Geometry: see drawing. Coordinates: mm, zero at the bounding-box minimum. A direction names the side the tool comes from. Round coordinates to 2 decimals unless told otherwise and drop trailing zeros. Write each loop counter-clockwise with the first axis right and the second up, starting at its lowest first coordinate (ties: lowest second). Pieces come first, ordered by that corner, then holes. Notation, with made-up numbers: (1.25, 89.5) -> (27.25, 89.5) arc R28 ccw to (27.25, 112.5) -> close; hole circle Ø1 at (58, 9). An arc over 180 degrees is marked (long way). Write item = value, one per line.
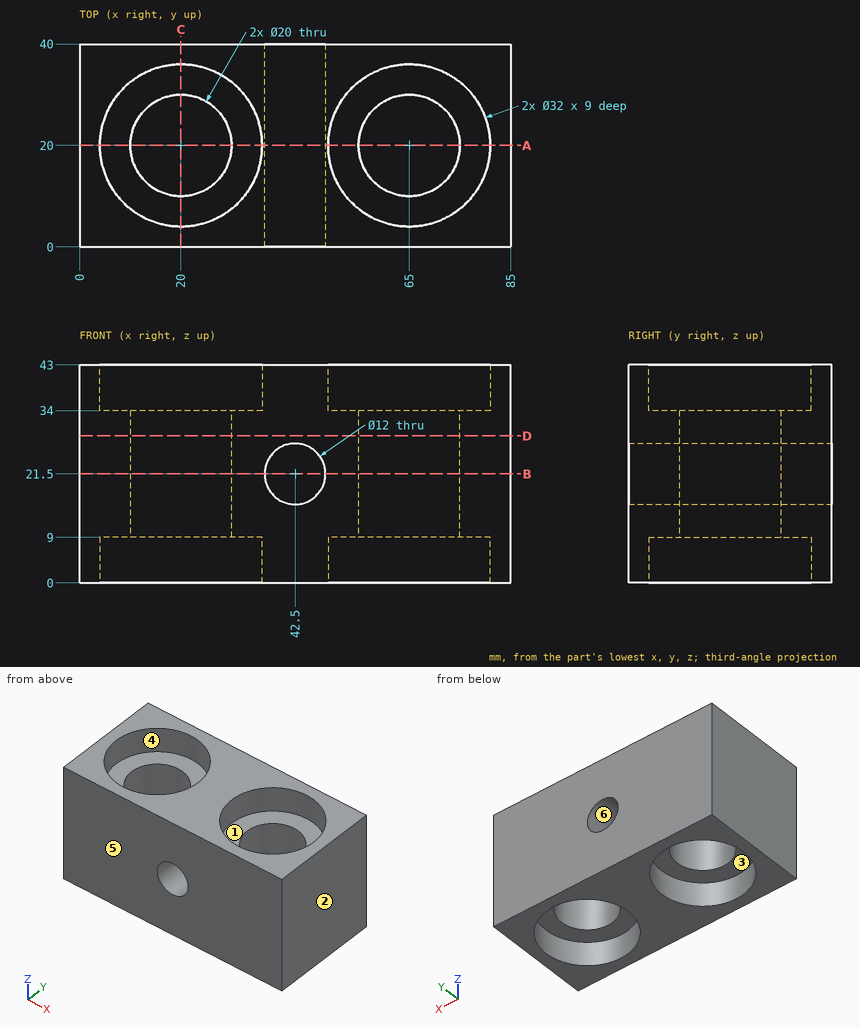
1) Cut plane B-B (z = 21.5). Return the cut outline in (x, y).
Solutions:
outline = (0, 0) -> (36.5, 0) -> (36.5, 40) -> (0, 40) -> close; (48.5, 0) -> (85, 0) -> (85, 40) -> (48.5, 40) -> close; hole circle Ø20 at (20, 20); hole circle Ø20 at (65, 20)
2) Cut plane A-A (y = 20). Count the separate pieces of the cut face and the enclosed holes in it, and give its area (3 significant figures).
Solutions:
separate_pieces = 3
enclosed_holes = 1
area = 1,390 mm^2
3) Cut plane D-D (z = 29). Return the cut outline in (x, y), and give its area (3 significant figures).
Solutions:
outline = (0, 0) -> (85, 0) -> (85, 40) -> (0, 40) -> close; hole circle Ø20 at (20, 20); hole circle Ø20 at (65, 20)
area = 2,770 mm^2
4) First-contact query: P1, Ø9.5, axis at x = 25, y = 24.5, coming from the +Z side; P2, Ø9.5, axis at x = 24.5, y = 16.5, coming from the -Z side. Flat tips, straight axial feed; report the tip coordinate or a pass-through.
Solutions:
P1 = 34
P2 = 9
5) Line query: L1, parallel to X at y = 20, z = 3.5; L2, parallel to X at y = 20, z = 22; L3, parallel to Y at x = 20, z = 6. Output: solid intervals per line, ascending. Write a range as from..to.
Solutions:
L1 = 0..4, 36..49, 81..85
L2 = 0..10, 30..36.52, 48.48..55, 75..85
L3 = 0..4, 36..40
6) Access query for the marked faces 1, 2 and 3. Directions: +Z, -Z, +X, -X, +Y, -Y. A direction counts if a zero-diameter tool reaches every point of the face in a straight line with its end or side. Return the directions, or none.
Solutions:
face_1 = +Z
face_2 = +Z, -Z, +X, +Y, -Y
face_3 = -Z
7) Cut plane C-C (x = 20). Return the cut outline in (y, z), and give its area (3 significant figures).
Solutions:
outline = (0, 0) -> (4, 0) -> (4, 9) -> (10, 9) -> (10, 34) -> (4, 34) -> (4, 43) -> (0, 43) -> close; (30, 9) -> (36, 9) -> (36, 0) -> (40, 0) -> (40, 43) -> (36, 43) -> (36, 34) -> (30, 34) -> close
area = 644 mm^2
8) Draft query along Y for the marked faces 4, 5 and 6. Return one class per face: +Y half, -Y half, draft (parallel to the pull), parting line (faces both ways), or undercut.
Solutions:
face_4 = undercut
face_5 = -Y half
face_6 = draft
